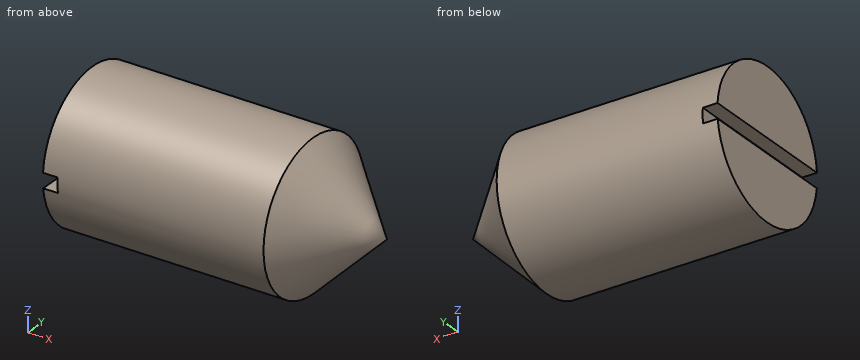
```python
from build123d import *

# Parameters (mm, degrees)
SKETCH1_W          = 7.62
SKETCH1_H          = 2.54
SKETCH2_W          = 0.508
SKETCH2_H          = 5.430732337
CUT_EXTRUDE1_DEPTH = 0.508


with BuildPart() as part:
    # Sketch1 → Revolve1 (revolve)
    with BuildSketch(Plane(origin=(0, 0, 0), x_dir=(1, 0, 0), z_dir=(0, 1, 0))):
        Polygon((7.62, -2.54), (10.16, -2.54), (7.62, 0), align=None)
        with Locations((3.81, -1.27)):
            Rectangle(SKETCH1_W, SKETCH1_H)
    revolve(axis=Axis((10.16, 0, 2.54), (-1, 0, 0)))

    # Sketch2 → Cut-Extrude1 (cut)
    with BuildSketch(Plane.ZY):
        with Locations((2.496486647, -0.018862031)):
            Rectangle(SKETCH2_W, SKETCH2_H)
    extrude(amount=-CUT_EXTRUDE1_DEPTH, mode=Mode.SUBTRACT)


solid = part.part
```
Read the model definition and answer for the solid it produces. Units are mm, in the model's axes. Coordinates: 2 decimals unless noted, no trailing zeros. Order: outer loops, then holes, each group sorted by start corner. A loop starts at its lowest first (then second) coordinate and runs counter-clockwise, first axis right, second up. Notation, with made-up numbers: (-15.5, 27) - (40.5, 27) arc R26 cw to (40.5, 56) - close; hole circle Ø3 at (81, 70.25). An arc over 180 degrees is marked (long way). Answer as a JSON object with one key per item and string values. Group by question number.
Item 1: Section A-A (x = 7.5) is taken. Give the vertices of the cut face in (y, z).
Item 2: Flat-ended cylindrical pins translate along their axes: P1, Ø0.6, axis at x = 0.5, y = 0.5, coming from the -Z side; P2, Ø0.6, axis at x = 0.5, y = -0.5, coming from the +Z side; P3, Ø1.5, axis at x = 8, z = 3.5, coming from the +Y side. Find the tip coordinate at first contact, or state that the pin passes through.
Item 3: Consider probe 1 along Y at (x, z) = (2, 2.3); probe 2 along X at (y, z) = (0.6, 3.25); probe 3 along Y at (x, z) = (9.75, 2.55). Determine where each line is inside the solid, lowest interval first. Write a range as from..to.
Results are:
{
 "1": {"outline": "circle Ø5.08 at (0, 2.54)"},
 "2": {"P1": "stops at z = 0.01", "P2": "stops at z = 5.07", "P3": "stops at y = 2.52"},
 "3": {"probe 1": "y = -2.53..2.53", "probe 2": "x = 0..9.23", "probe 3": "y = -0.41..0.41"}
}
